Autodesk Inventor part; units mm, degrees
ref_plane "YZ Plane" through (0, 0, 0) normal (1, 0, 0) x (0, 1, 0)
ref_plane "XZ Plane" through (0, 0, 0) normal (0, 1, 0) x (-1, 0, 0)
ref_plane "XY Plane" through (0, 0, 0) normal (0, 0, 1) x (1, 0, 0)
sketch "Sketch1" plane through (0, 0, 0) normal (0, 0, 1) x (1, 0, 0)
  line L0 (0, 0) -> (34, 0)
  line L1 (34, 0) -> (34, 11)
  line L2 (34, 11) -> (0, 11)
  line L3 (0, 11) -> (0, 0)
  circle A0 centre (17, 11) radius 11
  circle A1 centre (17, 11) radius 4
  line L4 (9.5554, 22) -> (24.3175, 22)
  point P0 (28, 11)
  point P1 (6, 11)
  dimension "d0" = 34
  dimension "d1" = 11
  dimension "d3" = 8
  dimension "d4" = 22
extrude "Extrusion1" add sketch "Sketch1" along normal blind 30 contours L3 L2 A0 L0 | A0 L2 L1 L0 | A0 L2 A1 | A0 L2 A1
sketch "Sketch2" plane through (0, 0, 0) normal (0, -1, 0) x (1, 0, 0)
  line L0 (34, 0) -> (34, 30)
  line L1 (0, 0) -> (0, 30)
  line L2 (0, 0) -> (34, 0)
  line L3 (0, 30) -> (34, 30)
  point P0 (5, 24)
  point P1 (29, 24)
  point P2 (29, 6)
  point P3 (5, 6)
  dimension "d7" = 24
  dimension "d8" = 18
  dimension "d9" = 5
  dimension "d10" = 5
  dimension "d11" = 6
  dimension "d12" = 6
hole "Hole1" at (5, 0, 24) at (29, 0, 24) at (29, 0, 6) at (5, 0, 6) direction (0, 1, 0) diameter 3.242 end through all
properties part number "Pillow block bearing"
Input: part model. Units: mm. Frame: model coordinates. A direction names the side the tool comes from. Coordinates: 2 decimals unless noted, no trailing zeros. Order: outer loops, then holes, each group sorted by start corner. A loop starts at its lowest first (then second) coordinate and runs counter-clockwise, first axis right, second up. Notation, with made-up numbers: M -36.75,-33.5 L 20.25,-33.5 A12 cw 20.25,-25.5 Z; hole C -5.5,62.5 d9. An arc over 180 degrees is marked long. Write item = value, one per line. Start each with the question number.
(1) First-contact query: P1, Ø6.5, axis at x = 2.5, z = 15.5, coming from the +Y side; P2, Ø4, axis at x = 8.5, z = 11.5, coming from the +Y side. Flat tips, straight axial feed; report the tip coordinate or a pass-through.
(2) Line query: line 1 along Z through (x, y) = (5, 9.75); line 2 along X through (y, z) = (6, 6); line 3 along Y through (x, z) = (17, 7.25). Output: solid intervals per line, ascending. Write a range as [from, to].
(3) Pull-direction query (Z, two-part tool) for faces 4 (the cylindrical face through (6.582, 5.798, 6.351)), 5 (the cylindrical face through (13.8, 13.4, 14.8)), 6 (the flat face through (17, 6, 0)); classes: released by +Z, released by -Z, zero draft, split by the parting line, or undercut.
(4) Section A-A on z = 24. Output: boundary loops of the cut face in (x, y).
(5) Section B-B on y = 9.5. Output: boundary loops of the cut face in (x, z).
(6) Reachability of faces 1 (the flat face through (17, 6, 30)), 2 (the flat face through (3, 11, 15)), 3 (the flat face through (31, 11, 15)) from +Z, -Z, +X, -X, +Y, -Y: full face, straight path, thin tool, end or side. Return the list, or none.
(7) Section C-C on x = 29. Output: boundary loops of the cut face in (y, z).
(8) Section D-D on y = 1.75. Output: boundary loops of the cut face in (x, z).
Result set:
q1.P1 = 11
q1.P2 = 19.87
q2.line_1 = [0, 4.38], [7.62, 22.38], [25.62, 30]
q2.line_2 = [0, 3.38], [6.62, 27.38], [30.62, 34]
q2.line_3 = [0, 7], [15, 22]
q3.face_4 = undercut
q3.face_5 = zero draft
q3.face_6 = released by -Z
q4.outline = M 0,0 L 3.38,0 L 3.38,11 L 0,11 Z; M 6.62,0 L 27.38,0 L 27.38,14.64 A11 ccw 6.62,14.64 Z; M 30.62,0 L 34,0 L 34,11 L 30.62,11 Z; hole C 17,11 d8
q5.outline = M 0,0 L 13.29,0 L 13.29,30 L 0,30 Z; M 20.71,0 L 34,0 L 34,30 L 20.71,30 Z; hole C 5,6 d3.24; hole C 5,24 d3.24; hole C 29,6 d3.24; hole C 29,24 d3.24
q6.face_1 = +Z, +X, -X, +Y, -Y
q6.face_2 = +Z, -Z, -X, +Y
q6.face_3 = +Z, -Z, +X, +Y
q7.outline = M 0,0 L 11,0 L 11,4.38 L 0,4.38 Z; M 0,7.62 L 11,7.62 L 11,22.38 L 0,22.38 Z; M 0,25.62 L 11,25.62 L 11,30 L 0,30 Z
q8.outline = M 0,0 L 34,0 L 34,30 L 0,30 Z; hole C 5,6 d3.24; hole C 5,24 d3.24; hole C 29,6 d3.24; hole C 29,24 d3.24
